Here's how the part is built. I have some questions about the finished solid (model axes, mm). Face numbers are marked on the shaded views. A direction names the side the tool comes from. Give positions to 0.01 mm unless a question says otherwise; leave off trailing zeros. Write each loop counter-clockwise with the first axis right and the second up, starting at its lowest first coordinate (ties: lowest second). Pieces come first, ordered by that corner, then holes. Notation, with made-up numbers: (22.25, -24.5) -> (54.25, -24.5) arc R16 ccw to (54.25, -12.5) -> close; hole circle Ø1 at (75, -23). An arc over 180 degrees is marked (long way). Use one line per item in the form item = value.
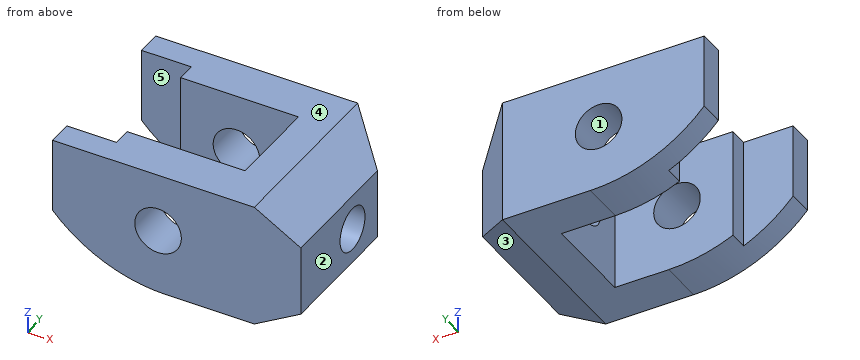
```python
from build123d import *

# Parameters (mm, degrees)
SKETCH1_R           = 7.5
BOSS_EXTRUDE1_DEPTH = 58
CUT_EXTRUDE1_DEPTH  = 58
CUT_EXTRUDE2_DEPTH  = 58
CUT_EXTRUDE3_REACH  = 82
SKETCH4_R           = 7


with BuildPart() as part:
    # Sketch1 → Boss-Extrude1 (new body)
    with BuildSketch(Plane(origin=(0, 0, 0), x_dir=(1, 0, 0), z_dir=(0, 1, 0))):
        with BuildLine():
            Line((36.66060556, 40), (65, 40))
            Line((65, 40), (80, 31.339745962))
            Line((80, 31.339745962), (80, 8.660254038))
            Line((80, 8.660254038), (65, 0))
            Line((65, 0), (0, 0))
            Line((0, 0), (0, 24))
            ThreePointArc((0, 24), (16.66060556, 35.82575695), (36.66060556, 40))
        make_face()
        with Locations((34, 19)):
            Circle(SKETCH1_R, mode=Mode.SUBTRACT)
    extrude(amount=BOSS_EXTRUDE1_DEPTH)

    # Sketch2 → Cut-Extrude1 (cut)
    with BuildSketch(Plane(origin=(0, 0, -40), x_dir=(-1, 0, 0), z_dir=(0, 0, -1))):
        Polygon((0, 50), (-16, 50), (-16, 44), (-54, 44), (-54, 14), (-16, 14), (-16, 8), (0, 8), align=None)
    extrude(amount=-CUT_EXTRUDE1_DEPTH, mode=Mode.SUBTRACT)

    # Sketch3 → Cut-Extrude2 (cut)
    with BuildSketch(Plane(origin=(0, 0, -40), x_dir=(-1, 0, 0), z_dir=(0, 0, -1))):
        Polygon((-80, 58), (-80, 43), (-65, 58), align=None)
    extrude(amount=-CUT_EXTRUDE2_DEPTH, mode=Mode.SUBTRACT)

    # Sketch4 → Cut-Extrude3 (cut, up to next)
    with BuildSketch(Plane(origin=(80, 0, 0), x_dir=(0, 0, -1), z_dir=(1, 0, 0)), mode=Mode.PRIVATE) as cut_extrude3_sk1:
        with Locations((20, 29)):
            Circle(SKETCH4_R)
    cut_extrude3_tool1 = extrude(cut_extrude3_sk1.sketch, amount=-CUT_EXTRUDE3_REACH, mode=Mode.PRIVATE) & part.part
    add(cut_extrude3_tool1.solids().sort_by_distance((80, 29, -20))[0], mode=Mode.SUBTRACT)


solid = part.part
```
Q1. Which directions (+Z, -Z, +X, -X, +Y, -Y) give clear straight access to the entire face, cutting with the end or side of a thin tool? Please do the marked faces 4 and 5.
Result set:
face_4 = +Z, +X, -X, +Y, -Y
face_5 = +Z, -Z, -X
Q2. I want a section at C-C, the plane x = 8. Write out the boundary of the cut face in (y, z).
Result set:
outline = (0, -30.97) -> (8, -30.97) -> (8, 0) -> (0, 0) -> close; (50, -30.97) -> (58, -30.97) -> (58, 0) -> (50, 0) -> close
Q3. If I drill on line 1 along Y through (x, z) = (59, -20); line 2 along Y through (x, z) = (42, -18); line 3 along X through (y, z) = (4, -19), over which ranges is the centre line in solid material (lowest first)? Write a range as from..to.
Result set:
line_1 = 0..22, 36..58
line_2 = 0..14, 44..58
line_3 = 0..26.5, 41.5..80
Q4. If we mould it in two halves opening along Z, with no side actions, what happens to the marked faces 1, 2 and 3? For each: +Z half, -Z half, draft (parallel to the pull), parting line (faces both ways), or undercut.
Result set:
face_1 = undercut
face_2 = draft
face_3 = -Z half
Q5. Will these pins go through, and if not, where does the flat tip stop? pin 1 Ø3 at (y, z) = (47, -17.5) entering from -X; pin 2 Ø6 at (x, y) = (18, 44.5) entering from +Z; pin 3 Ø6 at (y, z) = (32, -33.5) entering from -X.
Result set:
pin_1 = 16
pin_2 = 0
pin_3 = 54
Q6. I want a section at A-A, the plane y = 29. Write out the boundary of the cut face in (x, z).
Result set:
outline = (54, -40) -> (65, -40) -> (80, -31.34) -> (80, -27) -> (54, -27) -> close; (54, -13) -> (80, -13) -> (80, -8.66) -> (65, 0) -> (54, 0) -> close
Q7. I want a section at B-B, the plane z = -19. Write out the boundary of the cut face in (x, y).
Result set:
outline = (0, 0) -> (26.5, 0) -> (26.5, 14) -> (16, 14) -> (16, 8) -> (0, 8) -> close; (0, 50) -> (16, 50) -> (16, 44) -> (26.5, 44) -> (26.5, 58) -> (0, 58) -> close; (41.5, 0) -> (80, 0) -> (80, 22.07) -> (54, 22.07) -> (54, 14) -> (41.5, 14) -> close; (41.5, 44) -> (54, 44) -> (54, 35.93) -> (80, 35.93) -> (80, 43) -> (65, 58) -> (41.5, 58) -> close
Q8. I want a section at D-D, the plane x = 34. Write out the boundary of the cut face in (y, z), and give its area (3 significant figures).
Result set:
outline = (0, -39.93) -> (14, -39.93) -> (14, -26.5) -> (0, -26.5) -> close; (0, -11.5) -> (14, -11.5) -> (14, 0) -> (0, 0) -> close; (44, -39.93) -> (58, -39.93) -> (58, -26.5) -> (44, -26.5) -> close; (44, -11.5) -> (58, -11.5) -> (58, 0) -> (44, 0) -> close
area = 698 mm2
